Input: part model. Units: mm. Frame: model coordinates. Face numbers are marked on the shaded views. A direction names the side the tool comes from. Coordinates: 2 decimals unless noted, no trailing zeros. Write each loop counter-clockwise with the first axis right and the second up, starting at its lowest first coordinate (ties: lowest second). Pieces come first, ordered by that corner, then holes. Notation, with made-up numbers: (-40, 49) - (-24, 49) arc R12 ccw to (-24, 58) - close; hole circle Ø11 at (77.5, 73). An arc over 180 degrees is marked (long way). Put each result on its own line as item: value. Start each with the question number.
1. Cut plane A-A, the plane z = 35. Return loops of the section in (x, y), and give its area (3 significant figures).
2. Access query for the marked faces 1 and 2. Directions: +Z, -Z, +X, -X, +Y, -Y. A direction counts if a zero-diameter tool reaches every point of the face in a straight line with its end or side. Return the directions, or none.
3. Cut plane C-C, the plane y = 23. Return loops of the section in (x, z), and give its area (3 significant figures).
4. Pin query (flat end, axial travel): pin 1 (2 mm diameter, centred on x = -12, z = 7.5, fed in from +Y); pin 2 (1.5 mm diameter, centred on x = 21, y = 20, fed in from +Z); pin 3 (2 mm diameter, centred on y = -12, z = 41, fed in from +X); pin 4 (1 mm diameter, centred on x = -20, y = 22, fed in from +Z). Return the tip coordinate at first contact, or that it passes through.
5. Line query: line 1 (X direction, y = -12.5, z = 41.9); line 2 (Z direction, x = -12, y = 19.5); line 3 (Y direction, x = 2.5, z = 41.5). Output: solid intervals per line, ascending.
6. Cut plane B-B, the plane x = -6. Return loops of the section in (y, z), and give its area (3 significant figures).
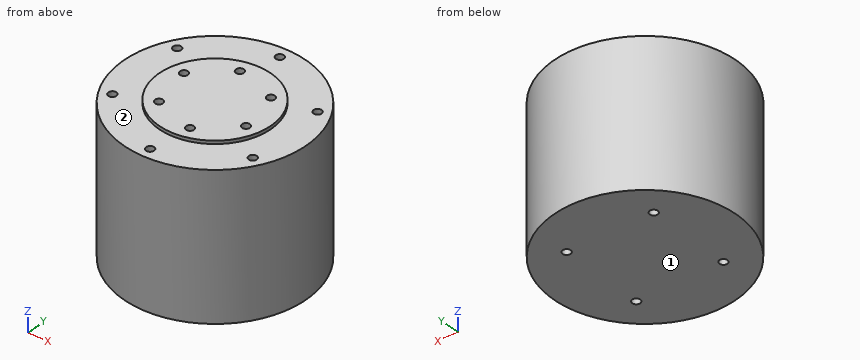
from build123d import *

# Parameters (mm, degrees)
SKETCH_1_R      = 28.5
EXTRUDE_1_DEPTH = 45
SKETCH_2_R      = 17.5
EXTRUDE_2_DEPTH = 1
M3X0_5_1_D      = 2.5
M3X0_5_1_DEPTH  = 4.248924226
M3X0_5_1_TIP    = 0.751075774
M3X0_5_2_D      = 2.5
M3X0_5_2_DEPTH  = 4.248924226
M3X0_5_2_TIP    = 0.751075774
M3X0_5_3_D      = 2.5
M3X0_5_3_DEPTH  = 4.248924226
M3X0_5_3_TIP    = 0.751075774


with BuildPart() as part:
    # 草图1 → 凸台-拉伸1 (new body)
    with BuildSketch(Plane.XY):
        with Locations(Location((0, 0, 0), (0, 0, 180))):
            Circle(SKETCH_1_R)
    extrude(amount=EXTRUDE_1_DEPTH)

    # 草图2 → 凸台-拉伸2 (add)
    with BuildSketch(Plane.XY.offset(45)):
        Circle(SKETCH_2_R)
    extrude(amount=EXTRUDE_2_DEPTH)

    # M3x0.5 螺纹孔1
    with Locations(Plane(origin=(0, 25, 45), x_dir=(1, 0, 0), z_dir=(0, 0, 1))):
        with Locations((0, 0), (21.650635095, -12.5), (21.650635095, -37.5), (0, -50), (-21.650635095, -37.5), (-21.650635095, -12.5)):
            Hole(M3X0_5_1_D / 2, depth=M3X0_5_1_DEPTH)
            with Locations((0, 0, -(M3X0_5_1_DEPTH + M3X0_5_1_TIP / 2))):  # 118° drill point
                Cone(0, M3X0_5_1_D / 2, M3X0_5_1_TIP, mode=Mode.SUBTRACT)

    # M3x0.5 螺纹孔2
    with Locations(Plane(origin=(-2.857682397, 13.194076372, 46), x_dir=(1, 0, 0), z_dir=(0, 0, 1))):
        with Locations((0, 0), (12.855246516, -4.122212634), (15.712928913, -17.316289006), (5.715364794, -26.388152744), (-7.139881722, -22.26594011), (-9.997564119, -9.071863738)):
            Hole(M3X0_5_2_D / 2, depth=M3X0_5_2_DEPTH)
            with Locations((0, 0, -(M3X0_5_2_DEPTH + M3X0_5_2_TIP / 2))):  # 118° drill point
                Cone(0, M3X0_5_2_D / 2, M3X0_5_2_TIP, mode=Mode.SUBTRACT)

    # M3x0.5 螺纹孔3
    with Locations(Plane(origin=(13.435028843, 13.435028843, 0), x_dir=(-1, 0, 0), z_dir=(0, 0, -1))):
        with Locations((0, 0), (0, -26.870057686), (26.870057686, -26.870057686), (26.870057686, 0)):
            Hole(M3X0_5_3_D / 2, depth=M3X0_5_3_DEPTH)
            with Locations((0, 0, -(M3X0_5_3_DEPTH + M3X0_5_3_TIP / 2))):  # 118° drill point
                Cone(0, M3X0_5_3_D / 2, M3X0_5_3_TIP, mode=Mode.SUBTRACT)


solid = part.part
Report:
1. outline: circle Ø57 at (0, 0)
1. area: 2,550 mm^2
2. face 1: -Z, +X, -X, +Y, -Y
2. face 2: +Z
3. outline: (-16.83, 0) - (16.83, 0) - (16.83, 45) - (-16.83, 45) - close
3. area: 1,510 mm^2
4. pin 1: stops at y = 26.29
4. pin 2: stops at z = 45
4. pin 3: stops at x = 26.29
4. pin 4: passes through
5. line 1: x = -25.61 to -22.9, -20.4 to 1.82, 3.9 to 20.4, 22.9 to 25.61
5. line 2: z = 0 to 45
5. line 3: y = -28.39 to -13.95, -12.44 to 28.39
6. outline: (-27.86, 0) - (27.86, 0) - (27.86, 45) - (16.44, 45) - (16.44, 46) - (-16.44, 46) - (-16.44, 45) - (-27.86, 45) - close
6. area: 2,540 mm^2
